Source: CAD feature listing. Evaluate the final solid. Frame: model axes, mm. Give positions to 0.01 mm unless a question says otherwise; leave off trailing zeros. Loops run counter-clockwise (first coordinate to the right, second up) from the corner with the lowest first, then second, coordinate; pieces in that order, holes last. Notation, with made-up numbers: M 58.5,42.25 L 99.5,42.25 A13 cw 99.5,56.25 Z; hole C -8.5,86 d7. An arc over 180 degrees is marked long. Answer in a Markdown table with one row per item.
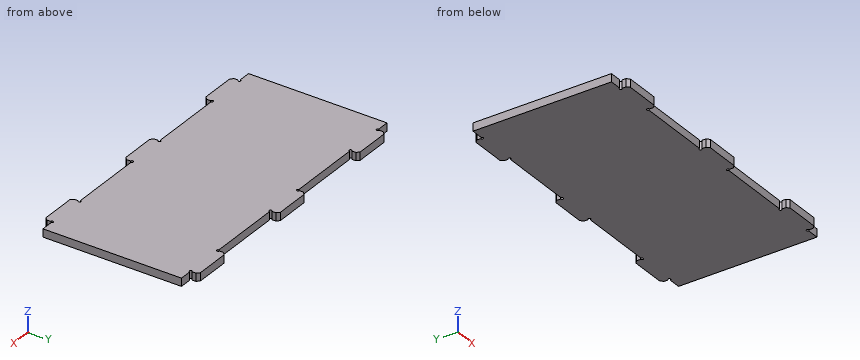
Autodesk Inventor part; units mm, degrees
ref_plane "Plan YZ" through (0, 0, 0) normal (1, 0, 0) x (0, 1, 0)
ref_plane "Plan XZ" through (0, 0, 0) normal (0, 1, 0) x (-1, 0, 0)
ref_plane "Plan XY" through (0, 0, 0) normal (0, 0, 1) x (1, 0, 0)
sketch "Esquisse7" plane through (0, 0, 0) normal (0, 0, 1) x (1, 0, 0)
  line L0 (-56.2, -26) -> (-56.2, 26)
  line L1 (-56.2, 26) -> (-51.2, 26)
  line L2 (-51.2, 26) -> (-51.2, 29)
  line L3 (-51.2, 29) -> (-36.2, 29)
  line L4 (-36.2, 29) -> (-36.2, 26)
  line L5 (36.2, 26) -> (36.2, 29)
  line L6 (36.2, 29) -> (51.2, 29)
  line L7 (51.2, 29) -> (51.2, 26)
  line L8 (51.2, 26) -> (56.2, 26)
  line L9 (56.2, 26) -> (56.2, -26)
  line L10 (56.2, -26) -> (51.2, -26)
  line L11 (51.2, -26) -> (51.2, -29)
  line L12 (51.2, -29) -> (36.2, -29)
  line L13 (36.2, -29) -> (36.2, -26)
  line L14 (-36.2, -26) -> (-36.2, -29)
  line L15 (-51.2, -29) -> (-51.2, -26)
  line L16 (-56.2, -26) -> (-51.2, -26)
  line L17 (-51.2, -29) -> (-36.2, -29)
  line L18 (0, -40.6) -> (0, 40.6) construction
  line L19 (-78.68, 0) -> (78.68, 0) construction
  line L20 (7.5, 26) -> (7.5, 29)
  line L21 (7.5, 29) -> (-7.5, 29)
  line L22 (-7.5, 29) -> (-7.5, 26)
  line L23 (7.5, -26) -> (7.5, -29)
  line L24 (7.5, -29) -> (-7.5, -29)
  line L25 (-7.5, -29) -> (-7.5, -26)
  line L26 (-36.2, -26) -> (-7.5, -26)
  line L27 (7.5, -26) -> (36.2, -26)
  line L28 (-36.2, 26) -> (-7.5, 26)
  line L29 (7.5, 26) -> (36.2, 26)
  point P0 (0, 0)
  dimension "d33" = 52
  dimension "d34" = 5
  dimension "d35" = 3
  dimension "d36" = 15
  dimension "d51" = 112.4
extrude "Extrusion2" add sketch "Esquisse7" along normal blind 3
chamfer "Chanfrein4" distance 1 angle 45 12 edges at (-51.2, 29, 1.5) (-7.5, 29, 1.5) (36.2, 29, 1.5) (-36.2, 29, 1.5) (7.5, 29, 1.5) (51.2, 29, 1.5) (-36.2, -29, 1.5) (-51.2, -29, 1.5) (-7.5, -29, 1.5) (7.5, -29, 1.5) (36.2, -29, 1.5) (51.2, -29, 1.5)
sketch "Esquisse9" plane through (0, 0, 3) normal (0, 0, 1) x (1, 0, 0)
  line L0 (-56.2, 26) -> (-51.2, 26) construction
  line L1 (-51.2, 26) -> (-51.2, 28) construction
  line L2 (-36.2, 28) -> (-36.2, 26) construction
  line L3 (-36.2, 26) -> (-7.5, 26) construction
  line L4 (-7.5, 26) -> (-7.5, 28) construction
  line L5 (7.5, 28) -> (7.5, 26) construction
  line L6 (7.5, 26) -> (36.2, 26) construction
  line L7 (36.2, 26) -> (36.2, 28) construction
  line L8 (51.2, 28) -> (51.2, 26) construction
  line L9 (51.2, 26) -> (56.2, 26) construction
  line L10 (7.5, -26) -> (7.5, -28) construction
  line L11 (36.2, -26) -> (7.5, -26) construction
  line L12 (36.2, -28) -> (36.2, -26) construction
  line L13 (51.2, -26) -> (51.2, -28) construction
  line L14 (56.2, -26) -> (51.2, -26) construction
  line L15 (-7.5, -26) -> (-36.2, -26) construction
  line L16 (-7.5, -28) -> (-7.5, -26) construction
  line L17 (-36.2, -26) -> (-36.2, -28) construction
  line L18 (-51.2, -28) -> (-51.2, -26) construction
  line L19 (-51.2, -26) -> (-56.2, -26) construction
  point P0 (0, 0)
hole "Perçage3" at (-51.2, 26, 3) at (-36.2, 26, 3) at (-7.5, 26, 3) at (36.2, 26, 3) at (51.2, 26, 3) at (7.5, 26, 3) at (36.2, -26, 3) at (51.2, -26, 3) at (7.5, -26, 3) at (-7.5, -26, 3) at (-36.2, -26, 3) at (-51.2, -26, 3) direction (0, 0, -1) diameter 1 end through all
properties part number "P1704_104" material "Plastique PMMA"
Q1. Contact query for flat-ended pins moving along their axis: pin 1 Ø0.8 at (y, z) = (27, 1.5) entering from -X; pin 2 Ø0.9 at (x, z) = (23, 1.5) entering from +Y; pin 3 Ø1.2 at (y, z) = (27, 2) entering from +X. Output: stop coordinate, or through.
Values follow:
| item | result |
|---|---|
| pin 1 | x = -51.2 |
| pin 2 | y = 26 |
| pin 3 | x = 51.2 |
Q2. Ray query, probe 1 along Y at (x, z) = (-16.5, 2.8); probe 2 along Y at (x, z) = (37, 2.15). Return the intervals inside material, ascending. Write a range as from..to.
Values follow:
| item | result |
|---|---|
| probe 1 | -26..26 |
| probe 2 | -28.8..28.8 |
Q3. Section query A-A (x = -25). Output: boundary loops of the cut face in (y, z).
Values follow:
| item | result |
|---|---|
| outline | M -26,0 L 26,0 L 26,3 L -26,3 Z |
